Autodesk Inventor part; units mm, degrees
ref_plane "YZ Plane" through (0, 0, 0) normal (1, 0, 0) x (0, 1, 0)
ref_plane "XZ Plane" through (0, 0, 0) normal (0, 1, 0) x (-1, 0, 0)
ref_plane "XY Plane" through (0, 0, 0) normal (0, 0, 1) x (1, 0, 0)
sketch "Sketch1" plane through (0, 0, 0) normal (0, 1, 0) x (-1, 0, 0)
  circle A0 centre (0, 0) radius 70
  dimension "d0" = 140
extrude "Extrusion1" add sketch "Sketch1" along normal blind 28
sketch "Sketch2" plane through (0, 28, 0) normal (0, 1, 0) x (1, 0, 0)
  circle A0 centre (0, 0) radius 8.25
  dimension "d3" = 16.5
extrude "Extrusion2" cut sketch "Sketch2" against normal blind 280
sketch "Sketch3" plane through (0, 28, 0) normal (0, 1, 0) x (1, 0, 0)
  circle A0 centre (0, 0) radius 8.25
  circle A1 centre (0, 0) radius 65
  circle A2 centre (0, 0) radius 10.5
  dimension "d6" = 130
  dimension "d7" = 21
extrude "Extrusion3" cut sketch "Sketch3" against normal blind 22 contours A1
sketch "Sketch4" plane through (0, 6, 0) normal (0, 1, 0) x (1, 0, 0)
  line L0 (-77.4845, 0) -> (88.5537, 0)
  line L1 (88.5537, 0) -> (88.5537, 100.8261)
  line L2 (88.5537, 100.8261) -> (-77.4845, 100.8261)
  line L3 (-77.4845, 100.8261) -> (-77.4845, 0)
  point P0 (0, 0)
extrude "Extrusion4" cut sketch "Sketch4" along normal blind 220
sketch "Sketch5" plane through (0, 0, 0) normal (0, -1, 0) x (1, 0, 0)
  circle A0 centre (0, 0) radius 8.25
  circle A1 centre (0, 0) radius 70
extrude "Extrusion5" cut sketch "Sketch5" against normal blind 3
sketch "Sketch6" plane through (0, 6, 0) normal (0, 1, 0) x (1, 0, 0)
  arc A0 (-65, 0) -> (65, 0) centre (0, 0) ccw
  line L0 (65, 0) -> (70, 0)
  arc A1 (70, 0) -> (-70, 0) centre (0, 0) ccw
  line L1 (-70, 0) -> (-65, 0)
  arc A2 (-10.5, 0) -> (10.5, 0) centre (0, 0) ccw
  line L2 (-10.5, 0) -> (-8.25, 0)
  arc A3 (8.25, 0) -> (-8.25, 0) centre (0, 0) ccw
  line L3 (8.25, 0) -> (10.5, 0)
  circle A4 centre (0, 0) radius 8.25
  arc A5 (65, 0) -> (-65, 0) centre (0, 0) ccw
  line L4 (-65, 0) -> (-70, 0)
  line L5 (65, 0) -> (70, 0)
  arc A6 (70, 0) -> (-70, 0) centre (0, 0) ccw
  arc A7 (70, 0) -> (70, 0) centre (0, 0) ccw
extrude "Extrusion6" cut sketch "Sketch6" against normal blind 3 contours L1 A1 L0 A5
sketch "Sketch7" plane through (0, 3, 0) normal (0, -1, 0) x (1, 0, 0)
  point P0 (0, 0)
sketch "Sketch8" plane through (0, 3, 0) normal (0, -1, 0) x (1, 0, 0)
  arc A0 (65, 0) -> (-65, 0) centre (0, 0) ccw
  arc A1 (70, 0) -> (-70, 0) centre (0, 0) ccw
  arc A2 (70, 0) -> (-70, 0) centre (0, 0) ccw
  arc A3 (65, 0) -> (-65, 0) centre (0, 0) ccw
  line L0 (65, 0) -> (70, 0)
  line L1 (70, 0) -> (65, 0)
  line L2 (-65, 0) -> (-70, 0)
  line L3 (-65, 0) -> (-70, 0)
extrude "Extrusion7" add sketch "Sketch8" along normal blind 3
sketch "Sketch9" plane through (0, 28, 0) normal (0, 1, 0) x (1, 0, 0)
  line L0 (10.5, 0) -> (-10.497, 0)
  line L1 (-10.497, 0) -> (-10.497, 68.6752)
  line L2 (-10.497, 68.6752) -> (10.5, 68.6752)
  line L3 (10.5, 68.6752) -> (10.5, 0)
  point P0 (0, 0)
extrude "Extrusion8" cut sketch "Sketch9" against normal blind 30
sketch "Sketch10" plane through (0, 3, 0) normal (0, -1, 0) x (1, 0, 0)
  arc A0 (8.25, 0) -> (-8.25, 0) centre (0, 0) ccw
  arc A1 (8.25, 0) -> (-8.25, 0) centre (0, 0) ccw
  line L0 (8.25, 0) -> (8.25, 64.4743)
  arc A2 (65, 0) -> (-65, 0) centre (0, 0) ccw
  line L1 (-8.25, 0) -> (-8.25, 64.4743)
  arc A3 (8.25, 64.4743) -> (-8.25, 64.4743) centre (0, 0) ccw
  point P0 (8.2498, 0.0514)
extrude "Extrusion9" add sketch "Sketch10" along normal blind 3
properties part number "casept1" material "PC/ABS Plastic"
Build history of the part. All positions in model axes, mm. A direction names the side the tool comes from. Coordinates: 2 decimals unless noted, no trailing zeros. Write each loop counter-clockwise with the first axis right and the second up, starting at its lowest first coordinate (ties: lowest second). Pieces come first, ordered by that corner, then holes. Notation, with made-up numbers: (-14.5, 54.25) -> (41.5, 54.25) arc R26 cw to (41.5, 81.25) -> close; hole circle Ø11 at (21, 76.5). An arc over 180 degrees is marked (long way). Use CSV: the item, a comma, the result in double quotes. Start each with the question number.
Q1. Flat gauge pins, fed straight in: pin 1 Ø10 at (y, z) = (15.5, 24.5) entering from -X; pin 2 Ø2.5 at (x, y) = (-68, 11) entering from -Z; pin 3 Ø3 at (x, y) = (-52.5, 10.5) entering from -Z. Where does each tip first touch, or does it go through?
Q2. Pull direction X, two halves, no side cores. Call faces 1 (the cylindrical face through (48.355, 1.521, 43.437)), 2 (the flat face through (0, 28, 66)), 3 (the cylindrical face through (1.539, 13.804, 69.983)), 4 (the flat face through (30, 3, 1)): released by +X, released by -X, zero draft, split by the parting line, or undercut.
Q3. 3-axis set-ups, long thin cutter, end or side, ignore diameter. For faces 5 (the cylindrical face through (-0.2, 17.2, 10.5)), 6 (the flat face through (10.5, 5, -33)), 7 (the flat face through (8.25, 2, 32)), 8 (the cylindrical face through (-49.12, 4.52, -42.57)), 9 (the flat face through (0, 0, 40)): which of +Z, -Z, +X, -X, +Y, -Y reach the whole face in a straight line?
Q4. Drill centre lines: probe 1 along Z at (x, y) = (0.5, 8.25); probe 2 along X at (y, z) = (17, 6.5); probe 3 along Y at (x, z) = (-62, 11). Where is each one in solid material? Low to high.
Q5. Cut at A-A, the plane y = 10.5. List the corners of the cut face in (x, z).
Q6. Cut at C-C, the plane z = -53. List the corners of the cut face in (x, y), then the cut area to 3 significant figures.
Q7. Cut at D-D, the plane z = 43. List the corners of the cut face in (x, y), then the cut area to 3 significant figures.
Q8. Cut at B-B, the plane x = 0. List the corners of the cut face in (y, z), then the cut area to 3 significant figures.
Checked values:
1,pin 1,"stops at x = -67.23"
1,pin 2,"stops at z = 0"
1,pin 3,"stops at z = 36.18"
2,face 1,"undercut"
2,face 2,"zero draft"
2,face 3,"split by the parting line"
2,face 4,"undercut"
3,face 5,"+Y"
3,face 6,"-Z, +Y, -Y"
3,face 7,"-Z, -Y"
3,face 8,"-Z, -X, +Y, -Y"
3,face 9,"+Z, -Z, +X, -X, -Y"
4,probe 1,"z = 8.23 to 10.49, 65 to 70"
4,probe 2,"x = -69.7 to -64.67, -8.25 to -5.08, 5.08 to 8.25, 64.67 to 69.7"
4,probe 3,"y = 3 to 6"
5,outline,"(-70, 0) -> (-65, 0) arc R65 cw to (65, 0) -> (70, 0) arc R70 ccw to start; (-10.5, 0) -> (-8.25, 0) arc R8.25 cw to (8.25, 0) -> (10.5, 0) arc R10.5 ccw to start"
6,outline,"(-37.63, 3) -> (-10.5, 3) -> (-10.5, 6) -> (-37.63, 6) -> close; (10.5, 3) -> (37.63, 3) -> (37.63, 6) -> (10.5, 6) -> close"
6,area,"163 mm²"
7,outline,"(-55.24, 0) -> (-48.74, 0) -> (-48.74, 3) -> (-8.25, 3) -> (-8.25, 0) -> (8.25, 0) -> (8.25, 3) -> (48.74, 3) -> (48.74, 0) -> (55.24, 0) -> (55.24, 28) -> (48.74, 28) -> (48.74, 6) -> (-48.74, 6) -> (-48.74, 28) -> (-55.24, 28) -> close"
7,area,"705 mm²"
8,outline,"(0, 8.25) -> (28, 8.25) -> (28, 10.5) -> (6, 10.5) -> (6, 65) -> (28, 65) -> (28, 70) -> (0, 70) -> close"
8,area,"530 mm²"
